Design review of the part built by this model. Coordinates are the model's own, in mm. A direction names the side the tool comes from. Round coordinates to 2 decimals unless told otherwise and drop trailing zeros. Order: outer loops, then holes, each group sorted by start corner. A loop starts at its lowest first (then second) coordinate and runs counter-clockwise, first axis right, second up. Notation, with made-up numbers: M 36,80.25 L 93,80.25 A21 ccw 93,99.25 Z; hole C 40,2.5 d11. An arc over 180 degrees is marked long. Use a Markdown table: item, result. Add a question column.
(1) To check wall thickness, follow probe 1 along Y at (x, z) = (-31, -14); probe 2 along X at (y, z) = (-26.5, -7.5). State the ranges of each line that lie inside material, in increasing order. Write a range as from..to.
(2) Take a section at C-C (y = -13.5). Write out the cut boundary in (x, z), then the cut area to 3 significant figures.
(3) Take a section at A-A (z = 11). Write out the cut boundary in (x, y) (3 decimals), then the cut area to 3 significant figures.
(4) Take a section at B-B (x = 6.5). Write out the cut boundary in (y, z).
(5) Take a section at D-D (x = 42). Write out the cut boundary in (y, z).
(6) For pin 1 (5 mm diameter, centred on x = -3.5, z = -35, fed in from -Y); pin 2 (2.5 mm diameter, centred on x = 47, z = 6.5, fed in from +Y) (3 decimals); pin 3 (7.5 mm diameter, centred on y = -33.5, z = 3, fed in from +X), all flat-tipped, find the tip position at first contact; note any pin that passes through.
(7) Machinability: for faces 1 (the face through (12.7, -25, 0)), 2 (the face through (0, -25, 12.7)), 3 (the face through (-12.7, -25, 0)), 4 (the face through (-47, 4.445, -1)), 5 (the face through (44.45, 6, -1)), which of the approach directions +Z, -Z, +X, -X, +Y, -Y give a long, thin tool a straight path to every point of the face, cutting with its end or side? Answer none if there is none.
```python
from build123d import *

# Parameters (mm, degrees)
SKETCH1_R           = 6.35
BOSS_EXTRUDE2_DEPTH = 7.62
SKETCH3_R           = 6.35
CUT_EXTRUDE2_DEPTH  = 3.175
SKETCH4_W           = 25.4
SKETCH4_H           = 25.4
BOSS_EXTRUDE3_DEPTH = 50.8
CUT_EXTRUDE4_DEPTH  = 102.6


with BuildPart() as part:
    # Sketch1 → Boss-Extrude2 (new body)
    with BuildSketch(Plane(origin=(0, 0, 0), x_dir=(1, 0, 0), z_dir=(0, 1, 0))):
        with BuildLine():
            Line((-69.85, 50.8), (69.85, 50.8))
            ThreePointArc((69.85, 50.8), (87.810512242, 43.360512242), (95.25, 25.4))
            Line((95.25, 25.4), (95.25, -25.4))
            ThreePointArc((95.25, -25.4), (87.810512242, -43.360512242), (69.85, -50.8))
            Line((69.85, -50.8), (-69.85, -50.8))
            ThreePointArc((-69.85, -50.8), (-87.810512242, -43.360512242), (-95.25, -25.4))
            Line((-95.25, -25.4), (-95.25, 25.4))
            ThreePointArc((-95.25, 25.4), (-87.810512242, 43.360512242), (-69.85, 50.8))
        make_face()
        with Locations((-69.85, 25.4)):
            Circle(SKETCH1_R, mode=Mode.SUBTRACT)
        with Locations((69.85, -25.4)):
            Circle(SKETCH1_R, mode=Mode.SUBTRACT)
        with Locations((69.85, 25.4)):
            Circle(SKETCH1_R, mode=Mode.SUBTRACT)
        with Locations((-69.85, -25.4)):
            Circle(SKETCH1_R, mode=Mode.SUBTRACT)
    extrude(amount=BOSS_EXTRUDE2_DEPTH)

    # Sketch3 → Cut-Extrude2 (cut)
    with BuildSketch(Plane(origin=(0, 7.62, 0), x_dir=(1, 0, 0), z_dir=(0, 1, 0))):
        with BuildLine():
            Line((-44.45, -50.8), (-44.45, 50.8))
            Line((-44.45, 50.8), (-69.85, 50.8))
            ThreePointArc((-69.85, 50.8), (-87.810512242, 43.360512242), (-95.25, 25.4))
            Line((-95.25, 25.4), (-95.25, -25.4))
            ThreePointArc((-95.25, -25.4), (-87.810512242, -43.360512242), (-69.85, -50.8))
            Line((-69.85, -50.8), (-44.45, -50.8))
        make_face()
        with Locations((-69.85, -25.4)):
            Circle(SKETCH3_R, mode=Mode.SUBTRACT)
        with Locations((-69.85, 25.4)):
            Circle(SKETCH3_R, mode=Mode.SUBTRACT)
        with BuildLine():
            Line((69.85, 50.8), (44.45, 50.8))
            Line((44.45, 50.8), (44.45, -50.8))
            Line((44.45, -50.8), (69.85, -50.8))
            ThreePointArc((69.85, -50.8), (87.810512242, -43.360512242), (95.25, -25.4))
            Line((95.25, -25.4), (95.25, 25.4))
            ThreePointArc((95.25, 25.4), (87.810512242, 43.360512242), (69.85, 50.8))
        make_face()
        with Locations((69.85, -25.4)):
            Circle(SKETCH3_R, mode=Mode.SUBTRACT)
        with Locations((69.85, 25.4)):
            Circle(SKETCH3_R, mode=Mode.SUBTRACT)
    extrude(amount=-CUT_EXTRUDE2_DEPTH, mode=Mode.SUBTRACT)

    # Sketch4 → Boss-Extrude3 (add)
    with BuildSketch(Plane.XZ):
        Rectangle(SKETCH4_W, SKETCH4_H)
    extrude(amount=BOSS_EXTRUDE3_DEPTH)

    # Sketch5 → Cut-Extrude4 (cut, through all)
    with BuildSketch(Plane.XY.offset(50.8)):
        Polygon((-49.53, 4.445), (-110.026455684, 4.445), (-110.026455684, 0), (-46.99, 0), align=None)
        Polygon((49.44093255, 4.445), (46.945466275, 0), (109.42401757, 0), (109.42401757, 4.445), align=None)
    extrude(amount=-CUT_EXTRUDE4_DEPTH, mode=Mode.SUBTRACT)


solid = part.part
```
Verdict:
| question | item | result |
|---|---|---|
| 1 | probe 1 | y = 0..7.62 |
| 1 | probe 2 | x = -12.7..12.7 |
| 2 | outline | M -12.7,-12.7 L 12.7,-12.7 L 12.7,12.7 L -12.7,12.7 Z |
| 2 | area | 645 mm^2 |
| 3 | outline | M -49.53,4.445 L -46.99,0 L -12.7,0 L -12.7,-50.8 L 12.7,-50.8 L 12.7,0 L 46.945,0 L 49.441,4.445 L 44.45,4.445 L 44.45,7.62 L -44.45,7.62 L -44.45,4.445 Z |
| 3 | area | 2,000 mm^2 |
| 4 | outline | M -50.8,-12.7 L 0,-12.7 L 0,-50.8 L 7.62,-50.8 L 7.62,50.8 L 0,50.8 L 0,12.7 L -50.8,12.7 Z |
| 5 | outline | M 0,-50.8 L 7.62,-50.8 L 7.62,50.8 L 0,50.8 Z |
| 6 | pin 1 | stops at y = 0 |
| 6 | pin 2 | stops at y = 4.445 |
| 6 | pin 3 | stops at x = 12.7 |
| 7 | face 1 | +Z, -Z, +X, -Y |
| 7 | face 2 | +Z, +X, -X, -Y |
| 7 | face 3 | +Z, -Z, -X, -Y |
| 7 | face 4 | +Z, -Z, -X, +Y |
| 7 | face 5 | +Z, -Z, +X, +Y |
